Check sheet for the modelled part. Datum: model origin and axes. Units: mm. Coordinates: 2 decimals unless noted, no trailing zeros. Order: outer loops, then holes, each group sorted by start corner. A loop starts at its lowest first (then second) coordinate and runs counter-clockwise, first axis right, second up.
1. Gauge pin test, flat ends, axial feed: pin 1 Ø1.5 at (x, z) = (-10, 1) entering from +Y; pin 2 Ø1.5 at (x, z) = (-3, 0) entering from +Y. Record the tip position at first contact, or that the pin passes through.
2. Cross-section at B-B (y = -105). Enter the section's corners in (x, z), then the cut area to 3 significant figures.
3. Thickness scan on line 1 (Z direction, x = -13.55, y = -10); line 2 (X direction, y = -103.5, z = 0); line 3 (Y direction, x = -10.25, z = 0.8). Record the ranges inside material, lowest first.
4. Cross-section at A-A (z = 0). Enter the section's corners in (x, y).
```python
from build123d import *

# Parameters (mm, degrees)
UTILITY_CIRCULAR_CROSS_SECTION_R   = 2
UTILITY_CIRCULAR_CROSS_SECTION_R_2 = 1.25


with BuildPart() as part:
    # Native hollow utility sweep: sweep along a path in Illustrative smooth utility route
    with BuildLine(Plane.XY) as native_hollow_utility_sweep_path:
        Line((-13.55, 0), (-13.55, -13.5))
        ThreePointArc((-13.55, -13.5), (-12.150414231, -19.152999757), (-8.275, -23.5))
        ThreePointArc((-8.275, -23.5), (-4.399585769, -27.847000243), (-3, -33.5))
        Line((-3, -33.5), (-3, -270.5))
    # Utility circular cross section → Native hollow utility sweep (sweep)
    with BuildSketch(Plane(origin=(0, 0, 0), x_dir=(1, 0, 0), z_dir=(0, 1, 0))):
        with Locations((-13.55, 0)):
            Circle(UTILITY_CIRCULAR_CROSS_SECTION_R)
        with Locations((-13.55, 0)):
            Circle(UTILITY_CIRCULAR_CROSS_SECTION_R_2, mode=Mode.SUBTRACT)
    sweep(path=native_hollow_utility_sweep_path.line)


solid = part.part
```
Data:
1. pin 1: stops at y = -17.89
1. pin 2: stops at y = -25.13
2. outline: circle Ø4 at (-3, 0); hole circle Ø2.5 at (-3, 0)
2. area: 7.66 mm2
3. line 1: z = -2 to -1.25, 1.25 to 2
3. line 2: x = -5 to -4.25, -1.75 to -1
3. line 3: y = -24.31 to -23.16, -20.34 to -18.79
4. outline: (-15.55, -13.5) arc R14.12 ccw to (-9.4, -25.15) arc R10.12 cw to (-5, -33.5) - (-5, -270.5) - (-4.25, -270.5) - (-4.25, -33.5) arc R10.87 ccw to (-8.98, -24.53) arc R13.37 cw to (-14.8, -13.5) - (-14.8, 0) - (-15.55, 0) - close; (-12.3, -13.5) arc R10.87 ccw to (-7.57, -22.47) arc R13.37 cw to (-1.75, -33.5) - (-1.75, -270.5) - (-1, -270.5) - (-1, -33.5) arc R14.12 ccw to (-7.15, -21.85) arc R10.12 cw to (-11.55, -13.5) - (-11.55, 0) - (-12.3, 0) - close
